Design review of the part built by this model. Coordinates are the model's own, in mm. Face numbers are marked on the shaded views. A direction names the side the tool comes from. Round coordinates to 2 decimals unless told otherwise and drop trailing zeros. Loops run counter-clockwise (first coordinate to the right, second up) from the corner with the lowest first, then second, coordinate; pieces in that order, holes last. Notation, with made-up numbers: M -29.75,55.25 L 11.25,55.25 A26 cw 11.25,71.25 Z; hole C 73.5,14.5 d10. An arc over 180 degrees is marked long. Use a Markdown table: item, result.
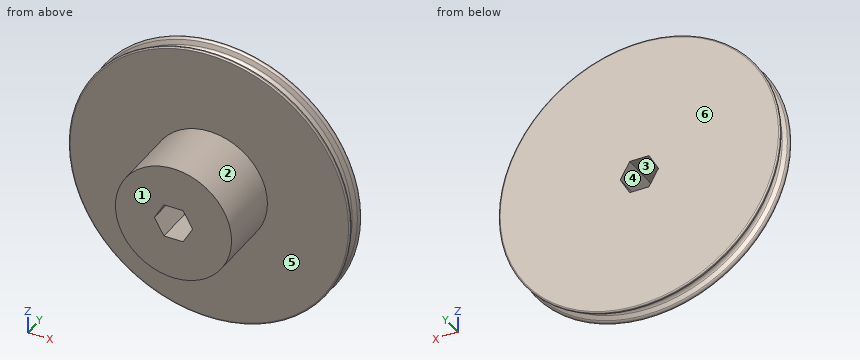
from build123d import *

# Parameters (mm, degrees)
CUT_EXTRUDE2_DEPTH  = 9.0000094
SKETCH3_R           = 22.225
BOSS_EXTRUDE1_DEPTH = 25.4


with BuildPart() as part:
    # Sketch1 → Revolve1 (revolve)
    with BuildSketch(Plane(origin=(0, 0, 0), x_dir=(0, 1, 0), z_dir=(0, 0, 1))):
        with BuildLine():
            Line((4.0000047, 0), (-4.0000047, 0))
            Line((-4.0000047, 0), (-4.0000047, 53.300621907))
            ThreePointArc((-4.0000047, 53.300621907), (-3.862299847, 53.645211447), (-3.525035946, 53.799994))
            ThreePointArc((-3.525035946, 53.799994), (-2.891173009, 53.65542644), (-2.425734949, 53.201499778))
            Line((-2.425734949, 53.201499778), (-1.558842609, 51.6999982))
            ThreePointArc((-1.558842609, 51.6999982), (0, 50.8), (1.558842609, 51.6999982))
            Line((1.558842609, 51.6999982), (2.425734949, 53.201499778))
            ThreePointArc((2.425734949, 53.201499778), (2.891173009, 53.65542644), (3.525035946, 53.799994))
            ThreePointArc((3.525035946, 53.799994), (3.862299847, 53.645211447), (4.0000047, 53.300621907))
            Line((4.0000047, 53.300621907), (4.0000047, 0))
        make_face()
    revolve(axis=Axis((0, 4.0000047, 0), (0, -1, 0)))

    # Sketch2 → Cut-Extrude2 (cut, through all)
    with BuildSketch(Plane.XZ.offset(4.0000047)):
        Polygon((7.332348419, 0), (3.666174209, 6.35), (-3.666174209, 6.35), (-7.332348419, 0), (-3.666174209, -6.35), (3.666174209, -6.35), align=None)
    extrude(amount=-CUT_EXTRUDE2_DEPTH, mode=Mode.SUBTRACT)

    # Sketch3 → Boss-Extrude1 (add)
    with BuildSketch(Plane.XZ.offset(4.0000047)):
        Circle(SKETCH3_R)
        Polygon((-3.666174209, 6.35), (-7.332348419, 0), (-3.666174209, -6.35), (3.666174209, -6.35), (7.332348419, 0), (3.666174209, 6.35), align=None, mode=Mode.SUBTRACT)
    extrude(amount=BOSS_EXTRUDE1_DEPTH)


solid = part.part
1. Take a section at B-B on y = 0. Give the boundary of the cut face in (x, z), and give its area (3 significant figures).
Check values:
| item | result |
|---|---|
| outline | C 0,0 d101.6; hole M -7.33,0 L -3.67,-6.35 L 3.67,-6.35 L 7.33,0 L 3.67,6.35 L -3.67,6.35 Z |
| area | 7,970 mm² |
2. Wall thickness on line 1 along Y through (x, z) = (-36, -14); line 2 along Z through (x, y) = (5, -12.5); line 3 along X through (y, z) = (-24, 8): over which ranges is each line inside the solid? List them lowest first. Write a range as from..to.
Check values:
| item | result |
|---|---|
| line 1 | y = -4..4 |
| line 2 | z = -21.66..-4.04, 4.04..21.66 |
| line 3 | x = -20.74..20.74 |
3. The part is to be moulded in two halves that separate along X. For the marked faces 1, 2 and 3, say which applies: pulls with the +X half, pulls with the -X half, needs draft (parallel to the pull), parting line crosses it, or undercut.
Check values:
| item | result |
|---|---|
| face 1 | needs draft |
| face 2 | parting line crosses it |
| face 3 | undercut |
4. Take a section at C-C on y = -19. Give the boundary of the cut face in (x, z) (3 decimals).
Check values:
| item | result |
|---|---|
| outline | C 0,0 d44.45; hole M -7.332,0 L -3.666,-6.35 L 3.666,-6.35 L 7.332,0 L 3.666,6.35 L -3.666,6.35 Z |
5. Insertion check: pin 1 (3.5 mm diameter, centred on x = -1, y = -9.5, fed in from -Z) (3 decimals); pin 2 (2 mm diameter, centred on x = -1.5, y = -13, fed in from +Z); pin 3 (8 mm diameter, centred on x = -43, y = -3.5, fed in from +Z). Each pin has a flat end and moves straight along its axis. Give the tip position at first contact, or say it passes through.
Check values:
| item | result |
|---|---|
| pin 1 | stops at z = -22.225 |
| pin 2 | stops at z = 22.22 |
| pin 3 | stops at z = 37.06 |
6. Machinability: for the marked faces 4, 5 and 6, which of the approach directions +Z, -Z, +X, -X, +Y, -Y give a long, thin tool a straight path to every point of the face, cutting with its end or side? Answer none if there is none.
Check values:
| item | result |
|---|---|
| face 4 | +Y, -Y |
| face 5 | -Y |
| face 6 | +Z, -Z, +X, -X, +Y |
